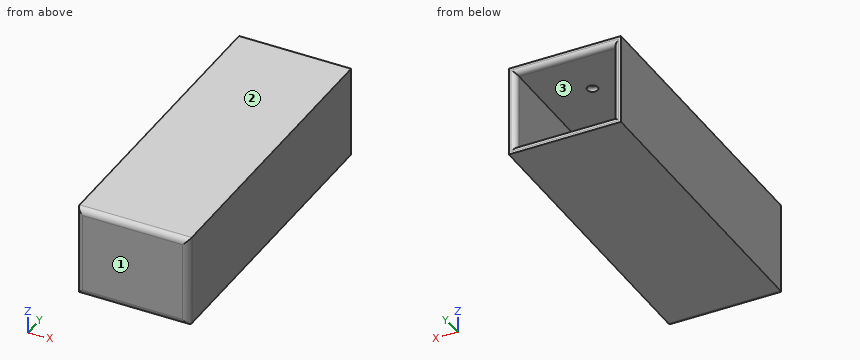
from build123d import *

# Parameters (mm, degrees)
F0_W      = 37.3
F0_H      = 30.4
F0_W_2    = 32.3
F0_H_2    = 25.4
F1_DEPTH  = 100
F2_W      = 37.3
F2_H      = 30.4
F3_DEPTH  = 3
F4_R      = 2
F5_R      = 1.75
F6_R      = 1.75
F7_DEPTH  = 1
F8_R      = 0.99999
F9_R      = 1.75
F10_DEPTH = 1
F11_R     = 0.99999
F12_W     = 32.3
F12_H     = 2
F13_DEPTH = 1
F14_W     = 32.3
F14_H     = 2
F15_DEPTH = 1


# Not quite as in the source:
# - a fillet or chamfer is up to 0.001 mm smaller than in the source, because OpenCascade refuses the exact size


with BuildPart() as f1:
    # F0 (on Front) → F1 (new body)
    with BuildSketch(Plane.XZ):
        with Locations((-0.3367068468, 2.3746712297)):
            Rectangle(F0_W, F0_H)
        with Locations((-0.3367068468, 2.3746712297)):
            Rectangle(F0_W_2, F0_H_2, mode=Mode.SUBTRACT)
    extrude(amount=F1_DEPTH)

    # F2 (on face) → F3 (join)
    with BuildSketch(Plane.XZ.offset(100)):
        with Locations((-0.3367068468, 2.3746712297)):
            Rectangle(F2_W, F2_H)
    extrude(amount=F3_DEPTH)

    # F4
    f4_edges = [f1.edges().sort_by_distance(p)[0] for p in [
        (-0.336707, -103, 17.574671),
        (-18.986707, -103, 2.374671),
        (-0.336707, -103, -12.825329),
        (18.313293, -103, 2.374671),
    ]]
    fillet(f4_edges, radius=F4_R)

    # F5
    f5_edges = [f1.edges().sort_by_distance(p)[0] for p in [
        (15.813293, 0, 2.374671),
        (-0.336707, 0, 15.074671),
        (-16.486707, 0, 2.374671),
        (-0.336707, 0, -10.325329),
    ]]
    fillet(f5_edges, radius=F5_R)

    # F6 (on face) → F7 (cut)
    with BuildSketch(Plane.XY.offset(-10.3253287703)):
        with Locations((-0.3367068468, -17.5)):
            Circle(F6_R)
    extrude(amount=-F7_DEPTH, mode=Mode.SUBTRACT)

    # F8 (radius 1 in the source; OpenCascade refuses exactly that, so slightly less here)
    f8_edges = [f1.edges().sort_by_distance(p)[0] for p in [
        (-2.086707, -17.5, -11.325329),
    ]]
    fillet(f8_edges, radius=F8_R)

    # F9 (on face) → F10 (cut)
    with BuildSketch(Plane(origin=(0, 0, 15.0746712297), x_dir=(1, 0, 0), z_dir=(0, 0, -1))):
        with Locations((-0.3367068468, 17.5)):
            Circle(F9_R)
    extrude(amount=-F10_DEPTH, mode=Mode.SUBTRACT)

    # F11 (radius 1 in the source; OpenCascade refuses exactly that, so slightly less here)
    f11_edges = [f1.edges().sort_by_distance(p)[0] for p in [
        (-2.086707, -17.5, 16.074671),
    ]]
    fillet(f11_edges, radius=F11_R)

    # F12 (on face) → F13 (join)
    with BuildSketch(Plane.XY.offset(-10.3253287703)):
        with Locations((-0.3367068468, -45.3)):
            Rectangle(F12_W, F12_H)
    extrude(amount=F13_DEPTH)

    # F14 (on face) → F15 (join)
    with BuildSketch(Plane(origin=(0, 0, 15.0746712297), x_dir=(1, 0, 0), z_dir=(0, 0, -1))):
        with Locations((-0.3367068468, 45.3)):
            Rectangle(F14_W, F14_H)
    extrude(amount=F15_DEPTH)


solid = f1.part
Build history of the part. All positions in model axes, mm. Face numbers are marked on the shaded views. Coordinates: 2 decimals unless noted, no trailing zeros. Order: outer loops, then holes, each group sorted by start corner. A loop starts at its lowest first (then second) coordinate and runs counter-clockwise, first axis right, second up. Notation, with made-up numbers: (-11, 58) -> (38, 58) arc R22 ccw to (38, 78) -> close; hole circle Ø8 at (21.25, 88.25). An arc over 180 degrees is marked (long way). One line per item, written item: value.
(1) Probe line 1 (X direction, y = -96, z = -7.5); line 2 (Z direction, x = 8, y = -91.5); line 3 (Y direction, x = -9, z = 15). List the from-to ranges inside material, lowest first. Write a range as [from, to].
Checked values:
line 1: [-18.99, -16.49], [15.81, 18.31]
line 2: [-12.83, -10.33], [15.07, 17.57]
line 3: [-103, -100], [-46.3, -44.3]
(2) Mould opens along Z. For the marked faces 1, 2 and 3 say: pulls with the +Z half, pulls with the -Z half, needs draft (parallel to the pull), parting line crosses it, or undercut.
Checked values:
face 1: needs draft
face 2: pulls with the +Z half
face 3: undercut
(3) Slice it at B-B, the plane x = -4.5. List the corners of the cut face in (y, z).
Checked values:
outline: (-103, -10.83) arc R2 ccw to (-101, -12.83) -> (0, -12.83) -> (0, -12.08) arc R1.75 ccw to (-1.75, -10.33) -> (-44.3, -10.33) -> (-44.3, -9.33) -> (-46.3, -9.33) -> (-46.3, -10.33) -> (-100, -10.33) -> (-100, 15.07) -> (-46.3, 15.07) -> (-46.3, 14.07) -> (-44.3, 14.07) -> (-44.3, 15.07) -> (-1.75, 15.07) arc R1.75 ccw to (0, 16.82) -> (0, 17.57) -> (-101, 17.57) arc R2 ccw to (-103, 15.57) -> close
(4) Drop flat-ended pins along their axis: pin 1 Ø7.5 at (x, z) = (-8, 8.5) entering from +Y; pin 2 Ø1 at (x, z) = (-10, 14.5) entering from +Y; pin 3 Ø1.1 at (x, z) = (3, -10) entering from +Y. Give the stop position or say it passes through.
Checked values:
pin 1: y = -100
pin 2: y = -44.3
pin 3: y = -0.89
(5) Slice it at C-C, the plane z = 12. List the corners of the cut face in (x, y).
Checked values:
outline: (-18.99, -101) arc R2 ccw to (-16.99, -103) -> (16.31, -103) arc R2 ccw to (18.31, -101) -> (18.31, 0) -> (17.56, 0) arc R1.75 ccw to (15.81, -1.75) -> (15.81, -100) -> (-16.49, -100) -> (-16.49, -1.75) arc R1.75 ccw to (-18.24, 0) -> (-18.99, 0) -> close
(6) Slice it at A-A, the plane y = -67.5. List the corners of the cut face in (x, z), plus the area to 4 significant figures.
Checked values:
outline: (-18.99, -12.83) -> (18.31, -12.83) -> (18.31, 17.57) -> (-18.99, 17.57) -> close; hole (-16.49, -10.33) -> (15.81, -10.33) -> (15.81, 15.07) -> (-16.49, 15.07) -> close
area: 313.5 mm2
